Check sheet for the modelled part. Datum: model origin and axes. Units: mm. A direction names the side the tool comes from. Round coordinates to 2 decimals unless told otherwise and drop trailing zeros.
Item 1: Go/stop test with flat-tipped pins: pin 1 Ø1.5 at (x, z) = (31, 3.5) entering from +Y; pin 2 Ø10 at (x, z) = (-18.5, -0.5) entering from -Y; pin 3 Ø3 at (x, z) = (8, 4.5) entering from +Y. Record where each tip stops, or that it passes through.
Item 2: Release check for a two-part mould opening along Y. For faces 1 (the flat face through (3.001, -47.897, 5.635)), 2 (the flat face through (6.151, -5.107, 12.074)) record: +Y half, -Y half, draft (parallel to the pull), parting line (faces both ways), or undercut.
Item 3: Tool access check on faces 3 (the flat face through (10.235, -38.867, 11.933)), 4 (the flat face through (-10.23, -31.62, 5.63)), 5 (the flat face through (3.72, -37.68, 12.07)). Record the directions out of +Z, -Z, +X, -X, +Y, -Y that give a thin tool (end or side, any length) a straight path to the whole face; none if there is none.
Item 4: Cross-section at A-A on z = 9. Count the separate pieces of the cut face and the enclosed holes in it, plus the area to 3 significant figures.
Item 5: Material ranges on line 1 (X direction, y = 13, z = 8.25); line 2 (X direction, y = 1, z = 0.25); line 3 (Y direction, x = 11, z = 10), recorded low to high.
from build123d import *

# Parameters (mm, degrees)
F1_R     = 50.8
F2_DEPTH = 6.35
F3_DEPTH = 12.7
F4_SIZE  = 1.27


with BuildPart() as f2:
    # F1 (on Top) → F2 (new body)
    with BuildSketch(Plane.XY):
        with Locations((0, -2.54)):
            Circle(F1_R)
    extrude(amount=-F2_DEPTH)

    # F0 (on Top) → F3 (join)
    with BuildSketch(Plane.XY):
        Polygon((-6.086908, -45.471568), (0, -50.254583), (0, -31.927135), (-2.555521, -29.379172), align=None)
        Polygon((-9.557882, -20.976724), (0, -27.727479), (0, 16.502708), (-9.268431, 16.502708), (-3.650971, 11.680054), align=None)
        Polygon((0, 16.502708), (0, -27.727479), (9.31712, -20.555755), (4.304654, 10.251204), (9.598721, 14.418875), (3.459856, 14.418875), (1.376021, 16.502708), align=None)
        Polygon((0, -31.927135), (0, -50.254583), (6.086908, -45.471568), (2.555521, -29.379172), align=None)
        Polygon((-9.457259, -4.413513), (-8.638233, 0), (-45.155544, 17.297892), (-41.290144, 10.121377), align=None)
        Polygon((-33.105214, -5.074794), (-29.343309, -12.059161), (-12.3377, -19.935444), (-11.434127, -15.066333), align=None)
        Polygon((-10.896486, -12.169126), (-10.012336, -7.404675), (-39.080556, 6.019047), (-35.312879, -0.976036), align=None)
        Polygon((-5.192886, -27.859336), (-7.740849, -25.937188), (-12.792072, -37.470073), (-8.366664, -41.001458), align=None)
        Polygon((8.638233, 0), (9.457259, -4.413513), (41.290144, 10.121377), (45.155544, 17.297892), align=None)
        Polygon((10.012336, -7.404675), (10.896486, -12.169126), (35.312879, -0.976036), (39.080556, 6.019047), align=None)
        Polygon((8.366664, -41.001458), (12.792072, -37.470073), (7.740849, -25.937188), (5.192886, -27.859336), align=None)
        Polygon((29.343309, -12.059161), (33.105214, -5.074794), (11.434127, -15.066333), (12.3377, -19.935444), align=None)
    extrude(amount=F3_DEPTH)

    # F4
    f4_edges = [f2.edges().sort_by_distance(p)[0] for p in [
        (-26.896888, 8.648946, 12.7),
        (-43.222844, 13.709634, 12.7),
        (-9.047746, -2.206757, 12.7),
        (-25.373702, 2.853932, 12.7),
        (-24.546446, -0.692814, 12.7),
        (-10.454411, -9.7869, 12.7),
        (-23.104682, -6.572581, 12.7),
        (-37.196717, 2.521506, 12.7),
        (-31.224262, -8.566978, 12.7),
        (-22.269671, -10.070563, 12.7),
        (-20.840504, -15.997303, 12.7),
        (-11.885913, -17.500888, 12.7),
        (9.047746, -2.206757, 12.7),
        (26.896888, 8.648946, 12.7),
        (25.373702, 2.853932, 12.7),
        (43.222844, 13.709634, 12.7),
        (10.454411, -9.7869, 12.7),
        (24.546446, -0.692814, 12.7),
        (23.104682, -6.572581, 12.7),
        (37.196717, 2.521506, 12.7),
        (11.885913, -17.500888, 12.7),
        (22.269671, -10.070563, 12.7),
        (31.224262, -8.566978, 12.7),
        (20.840504, -15.997303, 12.7),
        (-10.26646, -31.70363, 12.7),
        (-6.466867, -26.898262, 12.7),
        (-6.779775, -34.430397, 12.7),
        (-10.579368, -39.235765, 12.7),
        (-3.043454, -47.863076, 12.7),
        (3.043454, -47.863076, 12.7),
        (4.321215, -37.42537, 12.7),
        (-4.321215, -37.42537, 12.7),
        (-1.277761, -30.653154, 12.7),
        (1.277761, -30.653154, 12.7),
        (6.779775, -34.430397, 12.7),
        (6.466867, -26.898262, 12.7),
        (10.26646, -31.70363, 12.7),
        (10.579368, -39.235765, 12.7),
        (-4.778941, -24.352102, 12.7),
        (4.65856, -24.141617, 12.7),
        (-6.604427, -4.648335, 12.7),
        (6.810887, -5.152275, 12.7),
        (-6.459701, 14.091381, 12.7),
        (-3.946205, 16.502708, 12.7),
        (2.417938, 15.460792, 12.7),
        (6.529288, 14.418875, 12.7),
        (6.951687, 12.33504, 12.7),
        (-50.8, -2.54, 0),
    ]]
    chamfer(f4_edges, length=F4_SIZE)


solid = f2.part
Response values:
1. pin 1: stops at y = 10.95
1. pin 2: stops at y = -51.5
1. pin 3: stops at y = 14.42
2. face 1: -Y half
2. face 2: undercut
3. face 3: +Z, +X, -Y
3. face 4: +Z, -X
3. face 5: +Z
4. separate pieces: 10
4. enclosed holes: 0
4. area: 1,660 mm2
5. line 1: x = -42.84 to -36.08, -5.19 to 7.8, 36.08 to 42.84
5. line 2: x = -36.38 to -28.21, -21.31 to -10.75, -5.58 to 5.81, 10.75 to 21.31, 28.21 to 36.38
5. line 3: y = -38.9 to -33.38, -12.12 to -6.95, -3.71 to 1.12
